Work out the finished part from the listing and answer in its coordinate system (mm). A direction names the side the tool comes from. Coordinates: 2 decimals unless noted, no trailing zeros. Loops run counter-clockwise (first coordinate to the right, second up) from the corner with the lowest first, then second, coordinate; pieces in that order, holes last. Notation, with made-up numbers: (-4.5, 30) - (0.5, 30) arc R22 cw to (0.5, 46) - close; hole circle Ø6 at (-6.5, 67.25). An arc over 180 degrees is marked (long way). Write each question's results on one line, items separated by ' | '. Start each with the question number.
Item 1: Consider probe 1 along Z at (x, y) = (16.75, 0); probe 2 along Z at (x, y) = (14, -2); probe 3 along Y at (x, z) = (1.75, 15). Determine where each line is inside the solid, lowest interval first. Write a range as [from, to].
Item 2: Section C-C, the plane y = 15 is taken. Write down the section's boundary in (x, z), plus the area to 3 significant figures.
Item 3: Each of these flat-tipped pins is pushed along its axis until it touches: pin 1 Ø1 at (y, z) = (1.5, -16) entering from +X; pin 2 Ø6 at (y, z) = (14.5, -10.5) entering from +X; pin 3 Ø1.6 at (x, z) = (1, 16.5) entering from -Y; pin 4 Ø1.5 at (x, y) = (15, -19) entering from -Z. Where does it stop, or does it pass through?
Item 4: Section B-B, the plane x = 21 is taken. Write down the section's boundary in (y, z), plus the area to 3 significant figures.
Item 5: Section D-D, the plane z = -15 is taken. Write down the section's boundary in (x, y), plus the area to 3 significant figures.
Item 6: For a pull along Z with two mould halves and no side action, classify faces 4 (the face through (0, -2, 7)), 5 (the face through (15.21, 23.846, -7.509)), 6 (the face through (1, 2, 15)) as +Z half, -Z half, draft (parallel to the pull), parting line (faces both ways), or undercut.
Item 7: A tool of negligible diameter and unlimited length cuts with its end or side. For faces 1 (the face through (1, 0, 15)), 2 (the face through (2, 1, -15)), 3 (the face through (30, 4, 6)), from which of +Z, -Z, +X, -X, +Y, -Y can it reach the whole face along a straight path? Write none if from no direction.
Item 8: Section A-A, the plane z = 0 is taken. Write down the section's boundary in (x, y).
from build123d import *

# Parameters (mm, degrees)
ESBO_O1_W                = 30
ESBO_O1_H                = 25
ESBO_O2_R                = 7
CORTE_EXTRUS_O1_DEPTH    = 47.368092477
ESBO_O5_R                = 22
ESBO_O5_R_2              = 8
CORTE_EXTRUS_O3_DEPTH    = 47.368092477
ESBO_O6_W                = 15
ESBO_O6_H                = 2
RESSALTO_EXTRUS_O2_DEPTH = 2


with BuildPart() as part:
    # Esbo_o1 → Revolu_o1 (revolve)
    with BuildSketch(Plane.XY, mode=Mode.PRIVATE) as revolu_o1_sk:
        with Locations((15, -12.5)):
            Rectangle(ESBO_O1_W, ESBO_O1_H)
    revolve(revolu_o1_sk.sketch.rotate(Axis((30, 0, 0), (-1, 0, 0)), 180), axis=Axis((30, 0, 0), (-1, 0, 0)))

    # Esbo_o2 → Corte-extrus_o1 (cut, through all)
    with BuildSketch(Plane.ZY):
        Circle(ESBO_O2_R)
    extrude(amount=-CORTE_EXTRUS_O1_DEPTH, mode=Mode.SUBTRACT)

    # Esbo_o5 → Corte-extrus_o3 (cut, through all)
    with BuildSketch(Plane.ZY):
        with Locations(Location((0, 0, 0), (0, 0, 270))):
            Circle(ESBO_O5_R)
        with Locations(Location((0, 0, 0), (0, 0, 270))):
            Circle(ESBO_O5_R_2, mode=Mode.SUBTRACT)
    extrude(amount=-CORTE_EXTRUS_O3_DEPTH, mode=Mode.SUBTRACT)


with BuildPart() as corte_extrus_o3_piece_1:
    # of the separate pieces the step leaves, piece 1, a body of its own (corte_extrus_o3_pieces)
    add(part.part.solids().sort_by_distance((0, 25, 0))[0])



with BuildPart() as corte_extrus_o3_piece_2:
    # of the separate pieces the step leaves, piece 2, a body of its own (corte_extrus_o3_pieces)
    add(part.part.solids().sort_by_distance((0, -8, 0))[0])


with BuildPart() as corte_extrus_o3_piece_1_1:
    add(corte_extrus_o3_piece_1.part)

    add(corte_extrus_o3_piece_2.part)  # Ressalto-extrus_o2 merges Corte-extrus_o3 piece 2
    # Esbo_o6 → Ressalto-extrus_o2 (add)
    with BuildSketch(Plane.ZY):
        with Locations((-14.5, 1)):
            Rectangle(ESBO_O6_W, ESBO_O6_H)
        with Locations((14.5, 1)):
            Rectangle(ESBO_O6_W, ESBO_O6_H)
    extrude(amount=-RESSALTO_EXTRUS_O2_DEPTH)


solid = corte_extrus_o3_piece_1_1.part
Answer key:
1) probe 1: z = [-25, -22], [-8, -7], [7, 8], [22, 25] | probe 2: z = [-24.92, -21.91], [-7.75, -6.71], [6.71, 7.75], [21.91, 24.92] | probe 3: y = [-20, -16.09], [0, 2], [16.09, 20]
2) outline: (0, -20) - (30, -20) - (30, -16.09) - (0, -16.09) - close; (0, 16.09) - (30, 16.09) - (30, 20) - (0, 20) - close | area: 234 mm^2
3) pin 1: stops at x = 2 | pin 2: passes through | pin 3: stops at y = -19.46 | pin 4: stops at z = -17.09
4) outline: circle Ø50 at (0, 0); circle Ø16 at (0, 0); hole circle Ø44 at (0, 0); hole circle Ø14 at (0, 0) | area: 490 mm^2
5) outline: (0, -20) - (30, -20) - (30, -16.09) - (0, -16.09) - close; (0, 0) - (2, 0) - (2, 2) - (0, 2) - close; (0, 16.09) - (30, 16.09) - (30, 20) - (0, 20) - close | area: 238 mm^2
6) face 4: draft | face 5: parting line | face 6: undercut
7) face 1: +X, -X | face 2: +X | face 3: +Z, -Z, +X, +Y, -Y
8) outline: (0, -25) - (30, -25) - (30, -22) - (0, -22) - close; (0, -8) - (30, -8) - (30, -7) - (0, -7) - close; (0, 7) - (30, 7) - (30, 8) - (0, 8) - close; (0, 22) - (30, 22) - (30, 25) - (0, 25) - close
